Read the model definition and answer for the solid it produces. Units are mm, in the model's axes. Give positions to 0.01 mm unless a question says otherwise; leave off trailing zeros. Loops run counter-clockwise (first coordinate to the right, second up) from the corner with the lowest first, then second, coordinate; pieces in that order, holes last. Notation, with made-up numbers: (67.5, 8) - (113.5, 8) arc R19 ccw to (113.5, 23) - close; hole circle Ø3 at (-15.5, 54). An arc over 180 degrees is marked (long way). Use a Markdown table: item, result. Add a question column.
Item 1: A cutting plane is placed at B-B (y = -6.5). Determine the outline of the cut face in (x, z).
Item 2: A cutting plane is placed at C-C (z = -40.5). Determine the outline of the cut face in (x, y), plus the area to 3 significant figures.
Item 3: A cutting plane is placed at D-D (x = -24). Determine the outline of the cut face in (y, z), plus the area to 3 significant figures.
Item 4: A cutting plane is placed at A-A (x = 0). Determine the outline of the cut face in (y, z), plus the area to 3 significant figures.
Item 5: Each of these flat-tipped pins is pushed along its axis until it touches: P1, Ø6, axis at y = -7.5, z = -59.5, coming from the -X side; P2, Ø9, axis at x = -13.86, z = 52.64, coming from the -Y side; P3, Ø9, axis at x = 0, z = -53.43, coming from the -Y side; P4, Ø2, axis at y = -8.5, z = -60.5, coming from the -X side. Where does it stop, or does it pass through?
Item 6: Consider probe 1 along Z at (x, y) = (0, -7.25); probe 2 along Z at (x, y) = (-3.5, -3.75); probe 3 along X at (y, z) = (-12.5, 50.5). Determine where each line is inside the solid, lowest interval first. Write a range as [from, to].
Item 7: For a pull along Z with two mould halves and no side action, classify faces 1 (the face through (-29.863, -7, 25)), 2 (the face through (12.961, -12.146, 56.684)), 3 (the face through (13.339, -5.916, 56.603)), 4 (the face through (-13.9, -7.42, -74.93)) as +Z half, -Z half, draft (parallel to the pull), parting line (faces both ways), or undercut.
from build123d import *

# Parameters (mm, degrees)
PAD_DEPTH       = 15
CHAMFER_SIZE    = 2
SKETCH001_R     = 4
SKETCH001_R_2   = 5
POCKET_DEPTH    = 15.001
CHAMFER001_SIZE = 3


with BuildPart() as part:
    # Sketch → Pad (new body)
    with BuildSketch(Plane.XZ):
        Polygon((-29.863335, -15.849396), (-29.863335, 66.950175), (29.461527, 66.950175), (29.461527, -15.849396), (14.639226, -75.912064), (-14.639226, -75.912064), align=None)
    extrude(amount=PAD_DEPTH)

    # Chamfer
    chamfer_edges = [part.edges().sort_by_distance(p)[0] for p in [
        (-29.863335, -7.5, -15.849396),
        (-29.863335, -7.5, 66.950175),
        (-29.863335, 0, 25.55039),
        (-29.863335, -15, 25.55039),
        (29.461527, -7.5, 66.950175),
        (-0.200904, 0, 66.950175),
        (-0.200904, -15, 66.950175),
        (29.461527, -7.5, -15.849396),
        (29.461527, 0, 25.55039),
        (29.461527, -15, 25.55039),
        (14.639226, -7.5, -75.912064),
        (22.050376, 0, -45.88073),
        (22.050376, -15, -45.88073),
        (-14.639226, -7.5, -75.912064),
        (0, 0, -75.912064),
        (0, -15, -75.912064),
        (-22.251281, 0, -45.88073),
        (-22.251281, -15, -45.88073),
    ]]
    chamfer(chamfer_edges, length=CHAMFER_SIZE)

    # Sketch001 → Pocket (cut, through all)
    with BuildSketch(Plane.XZ):
        with Locations((-13.859818, 52.636753)):
            Circle(SKETCH001_R)
        with Locations((13.859818, 52.636753)):
            Circle(SKETCH001_R)
        with Locations((0, 32.020428)):
            Circle(SKETCH001_R)
        with Locations((0, -27.362068)):
            Circle(SKETCH001_R_2)
        with Locations((0, -53.42556)):
            Circle(SKETCH001_R_2)
    extrude(amount=POCKET_DEPTH, mode=Mode.SUBTRACT)

    # Chamfer001
    chamfer001_edges = [part.edges().sort_by_distance(p)[0] for p in [
        (-17.859818, -15, 52.636753),
        (9.859818, -15, 52.636753),
        (-4, -15, 32.020428),
    ]]
    chamfer(chamfer001_edges, length=CHAMFER001_SIZE)


solid = part.part
Geometry says:
| question | item | result |
|---|---|---|
| 1 | outline | (-29.86, -13.85) - (-29.37, -17.79) - (-15.13, -73.97) - (-12.64, -75.91) - (12.64, -75.91) - (15.12, -73.97) - (28.98, -17.79) - (29.46, -13.85) - (29.46, 64.95) - (27.46, 66.95) - (-27.86, 66.95) - (-29.86, 64.95) - close; hole circle Ø8 at (-13.86, 52.64); hole circle Ø10 at (0, -53.43); hole circle Ø10 at (0, -27.36); hole circle Ø8 at (0, 32.02); hole circle Ø8 at (13.86, 52.64) |
| 2 | outline | (-23.62, -13) - (-21.55, -15) - (21.32, -15) - (23.38, -13) - (23.38, -2) - (21.32, 0) - (-21.55, 0) - (-23.62, -2) - close |
| 2 | area | 697 mm² |
| 3 | outline | (-15, -30.84) - (-13, -38.98) - (-2, -38.98) - (0, -30.84) - (0, 64.95) - (-2, 66.95) - (-13, 66.95) - (-15, 64.95) - close |
| 3 | area | 1,570 mm² |
| 4 | outline | (-15, -73.91) - (-13, -75.91) - (-2, -75.91) - (0, -73.91) - (0, -58.43) - (-15, -58.43) - close; (-15, -48.43) - (0, -48.43) - (0, -32.36) - (-15, -32.36) - close; (-15, -22.36) - (0, -22.36) - (0, 28.02) - (-12, 28.02) - (-15, 25.02) - close; (-15, 39.02) - (-12, 36.02) - (0, 36.02) - (0, 64.95) - (-2, 66.95) - (-13, 66.95) - (-15, 64.95) - close |
| 4 | area | 1,710 mm² |
| 5 | P1 | x = -19.56 |
| 5 | P2 | y = -12.5 |
| 5 | P3 | through |
| 5 | P4 | x = -18.8 |
| 6 | probe 1 | [-75.91, -58.43], [-48.43, -32.36], [-22.36, 28.02], [36.02, 66.95] |
| 6 | probe 2 | [-75.91, -57], [-49.85, -30.93], [-23.79, 30.08], [33.96, 66.95] |
| 6 | probe 3 | [-29.86, -17.82], [-9.9, 9.9], [17.82, 29.46] |
| 7 | face 1 | draft |
| 7 | face 2 | undercut |
| 7 | face 3 | undercut |
| 7 | face 4 | -Z half |
